Could you check a few things on this model? Use its own coordinates, in mm. Face numbers are marked on the shaded views. Round coordinates to 2 decimals unless told otherwise and drop trailing zeros. Loops run counter-clockwise (first coordinate to the right, second up) from the corner with the lowest first, then second, coordinate; pieces in that order, holes last. Notation, with made-up numbers: (64, -14) -> (107, -14) arc R19 ccw to (107, 3) -> close; hole circle Ø2 at (-18.5, -10). An arc over 180 degrees is marked (long way). Write each question's results on one line, items separated by ' | '. Start each with the question number.
1) Imagine slicing it at B-B, the plane x = -20.75. List the corners of the cut face in (y, z) for me (3 decimals), plus the area to 3 significant figures.
2) For P1, Ø12, axis at x = -10.5, z = 11.5, coming from the -Y side; P2, Ø3.5, axis at x = -20.75, z = -15.25, coming from the +Y side, each with a flat end and sliding along its axis, tell me the tip position at first contact or that it passes through.
3) Imagine slicing it at D-D, the plane x = -1. List the corners of the cut face in (y, z) for me (3 decimals), plus the area to 3 significant figures.
4) We'd pull the mould along Z, two halves only. Please class the marked faces 1, 2 and 3: pulls with the +Z half, pulls with the -Z half, needs draft (parallel to the pull), parting line crosses it, or undercut.
5) If I drill on probe 1 along X at (y, z) = (19, 15.25) (3 decimals); probe 2 along Z at (x, y) = (-20.75, 22.75) (3 decimals); probe 3 along Z at (x, y) = (20.75, 24) (3 decimals), over which ranges is the centre line in solid material (lowest first)?
6) Imagine slicing it at C-C, the plane z = 15.25. List the corners of the cut face in (x, y) for me (3 decimals), plus the area to 4 significant figures.
7) Imagine slicing it at A-A, the plane y = 19.5. List the corners of the cut face in (x, z) for me (3 decimals).
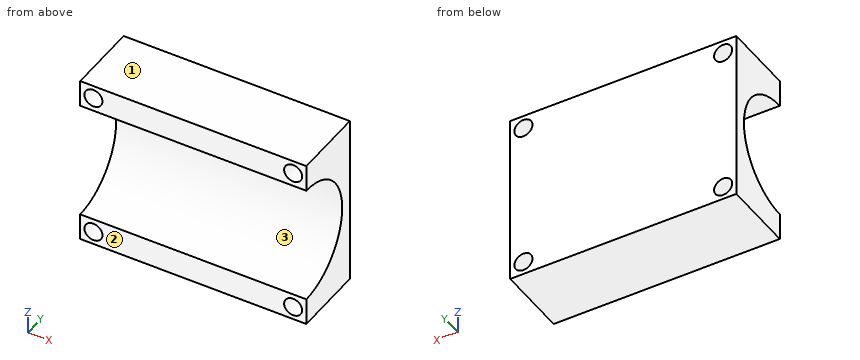
from build123d import *

# Parameters (mm, degrees)
SKETCH1_W           = 47
SKETCH1_H           = 36
BOSS_EXTRUDE1_DEPTH = 30
SKETCH3_R           = 12.375
CUT_EXTRUDE1_DEPTH  = 47
SKETCH5_R           = 1.875
CUT_EXTRUDE2_DEPTH  = 40
CUT_EXTRUDE3_START  = 23.5
SKETCH7_W           = 36
SKETCH7_H           = 15
CUT_EXTRUDE3_DEPTH  = 48


with BuildPart() as part:
    # Sketch1 → Boss-Extrude1 (new body)
    with BuildSketch(Plane(origin=(0, 0, 0), x_dir=(1, 0, 0), z_dir=(0, 1, 0))):
        Rectangle(SKETCH1_W, SKETCH1_H)
    extrude(amount=BOSS_EXTRUDE1_DEPTH)

    # Sketch3 → Cut-Extrude1 (cut)
    with BuildSketch(Plane(origin=(23.5, 0, 0), x_dir=(0, 0, -1), z_dir=(1, 0, 0))):
        with Locations((0, 15)):
            Circle(SKETCH3_R)
    extrude(amount=-CUT_EXTRUDE1_DEPTH, mode=Mode.SUBTRACT)

    # Sketch5 → Cut-Extrude2 (cut)
    with BuildSketch(Plane(origin=(0, 30, 0), x_dir=(1, 0, 0), z_dir=(0, 1, 0))):
        with Locations((-20.75, 15.25)):
            Circle(SKETCH5_R)
        with Locations((-20.75, -15.25)):
            Circle(SKETCH5_R)
        with Locations((20.75, -15.25)):
            Circle(SKETCH5_R)
        with Locations((20.75, 15.25)):
            Circle(SKETCH5_R)
    extrude(amount=-CUT_EXTRUDE2_DEPTH, mode=Mode.SUBTRACT)

    # Sketch7 → Cut-Extrude3 (cut, through all)
    with BuildSketch(Plane(origin=(0, 0, 0), x_dir=(0, 0, -1), z_dir=(1, 0, 0)).offset(CUT_EXTRUDE3_START)):
        with Locations((0, 7.5)):
            Rectangle(SKETCH7_W, SKETCH7_H)
    extrude(amount=-CUT_EXTRUDE3_DEPTH, mode=Mode.SUBTRACT)


solid = part.part
Checked values:
1) outline: (15, -18) -> (30, -18) -> (30, -17.125) -> (15, -17.125) -> close; (15, -13.375) -> (30, -13.375) -> (30, 13.375) -> (15, 13.375) -> (15, 12.375) arc R12.375 cw to (15, -12.375) -> close; (15, 17.125) -> (30, 17.125) -> (30, 18) -> (15, 18) -> close | area: 187 mm^2
2) P1: y = 15 | P2: through
3) outline: (15, -18) -> (30, -18) -> (30, 18) -> (15, 18) -> (15, 12.375) arc R12.375 cw to (15, -12.375) -> close | area: 299 mm^2
4) face 1: pulls with the +Z half | face 2: needs draft | face 3: undercut
5) probe 1: -23.5 to -22.625, -18.875 to 18.875, 22.625 to 23.5 | probe 2: -18 to -17.125, -13.375 to -9.648, 9.648 to 13.375, 17.125 to 18 | probe 3: -18 to -17.125, -13.375 to -8.494, 8.494 to 13.375, 17.125 to 18
6) outline: (-23.5, 15) -> (-22.625, 15) -> (-22.625, 30) -> (-23.5, 30) -> close; (-18.875, 15) -> (18.875, 15) -> (18.875, 30) -> (-18.875, 30) -> close; (22.625, 15) -> (23.5, 15) -> (23.5, 30) -> (22.625, 30) -> close | area: 592.5 mm^2
7) outline: (-23.5, -18) -> (23.5, -18) -> (23.5, -11.528) -> (-23.5, -11.528) -> close; (-23.5, 11.528) -> (23.5, 11.528) -> (23.5, 18) -> (-23.5, 18) -> close; hole circle Ø3.75 at (-20.75, -15.25); hole circle Ø3.75 at (-20.75, 15.25); hole circle Ø3.75 at (20.75, -15.25); hole circle Ø3.75 at (20.75, 15.25)
